```python
from build123d import *

# Parameters (mm, degrees)
SKETCH1_R           = 2.5
BOSS_EXTRUDE1_DEPTH = 23
BOSS_EXTRUDE2_DEPTH = 3
BOSS_EXTRUDE3_DEPTH = 3
BOSS_EXTRUDE4_START = 2
SKETCH4_R           = 2.5
BOSS_EXTRUDE4_DEPTH = 2


with BuildPart() as part:
    # Sketch1 → Boss-Extrude1 (new body)
    with BuildSketch(Plane.XY):
        Circle(SKETCH1_R)
    extrude(amount=BOSS_EXTRUDE1_DEPTH)

    # Sketch2 → Boss-Extrude2 (add)
    with BuildSketch(Plane.XY.offset(23)):
        Polygon((2.489504252, 3.890462943), (-2.124487616, 4.101205397), (-4.613991867, 0.210742453), (-2.489504252, -3.890462943), (2.124487616, -4.101205397), (4.613991867, -0.210742453), align=None)
    extrude(amount=BOSS_EXTRUDE2_DEPTH)

    # Sketch3 → Boss-Extrude3 (add)
    with BuildSketch(Plane(origin=(0, 0, 0), x_dir=(-1, 0, 0), z_dir=(0, 0, -1))):
        Polygon((4.077074227, 2.170437533), (0.158883072, 4.61606862), (-3.918191154, 2.445631087), (-4.077074227, -2.170437533), (-0.158883072, -4.61606862), (3.918191154, -2.445631087), align=None)
    extrude(amount=-BOSS_EXTRUDE3_DEPTH)

    # Sketch4 → Boss-Extrude4 (add)
    with BuildSketch(Plane(origin=(0, 0, 0), x_dir=(-1, 0, 0), z_dir=(0, 0, -1)).offset(BOSS_EXTRUDE4_START)):
        Circle(SKETCH4_R)
    extrude(amount=-BOSS_EXTRUDE4_DEPTH)


solid = part.part
```
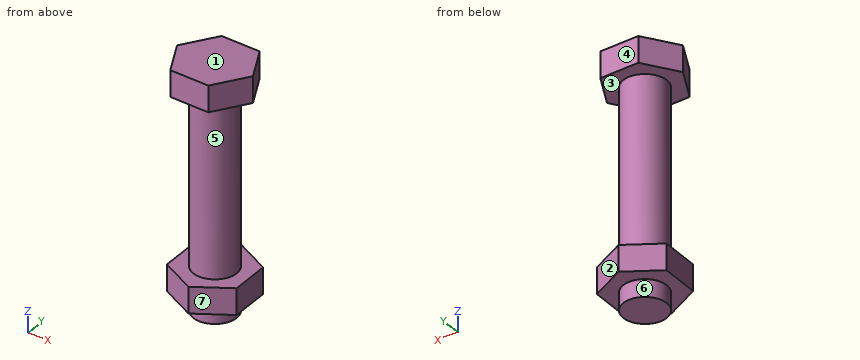
Geometry: final body of the model. Coordinates: model frame, mm. Face numbers are marked on the shaded views. A direction names the side the tool comes from. Round coordinates to 2 decimals unless told otherwise and drop trailing zeros. Order: outer loops, then holes, each group sorted by start corner. A loop starts at its lowest first (then second) coordinate and runs counter-clockwise, first axis right, second up. Notation, with made-up numbers: (-3.75, 14) -> (3.25, 14) arc R14 ccw to (3.25, 31) -> close; hole circle Ø7 at (50.5, 30.5). An arc over 180 degrees is marked (long way). Use CSV: the item, a comma, the result in double quotes. Start each with the question number.
1) Set-up query: the marked faces 4, 5, 6 and 7. Return all of +Z, -Z, +X, -X, +Y, -Y with unobstructed straight access to the full face (end or side cutting, diameter ignored); none if empty.
2) First-contact query: pin 1 Ø1.5 at (x, y) = (-3.5, 1.5) entering from -Z; pin 2 Ø4 at (x, z) = (-3, 22) entering from -Y; pin 3 Ø3 at (x, z) = (-2, 17.5) entering from -Y. Flat tips, straight axial feed; report the tip coordinate or a pass-through.
3) Material intervals for line 1 along Z through (x, y) = (0, -2.75); line 2 along X through (y, z) = (0.25, 17); line 3 along Z through (x, y) = (4, -1.5), sorted ascending. Write a range as from..to.
4) Section D-D (y = -1). Return the cut outline in (x, z).
5) Section B-B (x = -3.5). Return the cut outline in (y, z).
6) Section C-C (z = 2). Return the cut outline in (x, y), and give its area (3 significant figures).
7) Section A-A (y = -3). Return the cut outline in (x, z).
8) Draft query along Z for the marked faces 1, 2 and 3. Return one class per face: +Z half, -Z half, draft (parallel to the pull), parting line (faces both ways), or undercut.
Returned:
1,face 4,"+Z, +X, +Y"
1,face 5,"none"
1,face 6,"-Z"
1,face 7,"-Z, +X, -Y"
2,pin 1,"stops at z = 0"
2,pin 2,"stops at y = -3.95"
2,pin 3,"stops at y = -2.45"
3,line 1,"z = 0..3, 23..26"
3,line 2,"x = -2.49..2.49"
3,line 3,"z = 0..3"
4,outline,"(-3.99, 23) -> (-2.29, 23) -> (-2.29, 3) -> (-3.97, 3) -> (-3.97, 0) -> (-2.29, 0) -> (-2.29, -2) -> (2.29, -2) -> (2.29, 0) -> (4.04, 0) -> (4.04, 3) -> (2.29, 3) -> (2.29, 23) -> (4.11, 23) -> (4.11, 26) -> (-3.99, 26) -> close"
5,outline,"(-2.67, 0) -> (2.53, 0) -> (2.53, 3) -> (-2.67, 3) -> close; (-1.94, 23) -> (1.95, 23) -> (1.95, 26) -> (-1.94, 26) -> close"
6,outline,"(-4.08, 2.17) -> (-3.92, -2.45) -> (0.16, -4.62) -> (4.08, -2.17) -> (3.92, 2.45) -> (-0.16, 4.62) -> close"
6,area,"55.4 mm²"
7,outline,"(-2.95, 23) -> (2.83, 23) -> (2.83, 26) -> (-2.95, 26) -> close; (-2.88, 0) -> (2.75, 0) -> (2.75, 3) -> (-2.88, 3) -> close"
8,face 1,"+Z half"
8,face 2,"draft"
8,face 3,"undercut"
